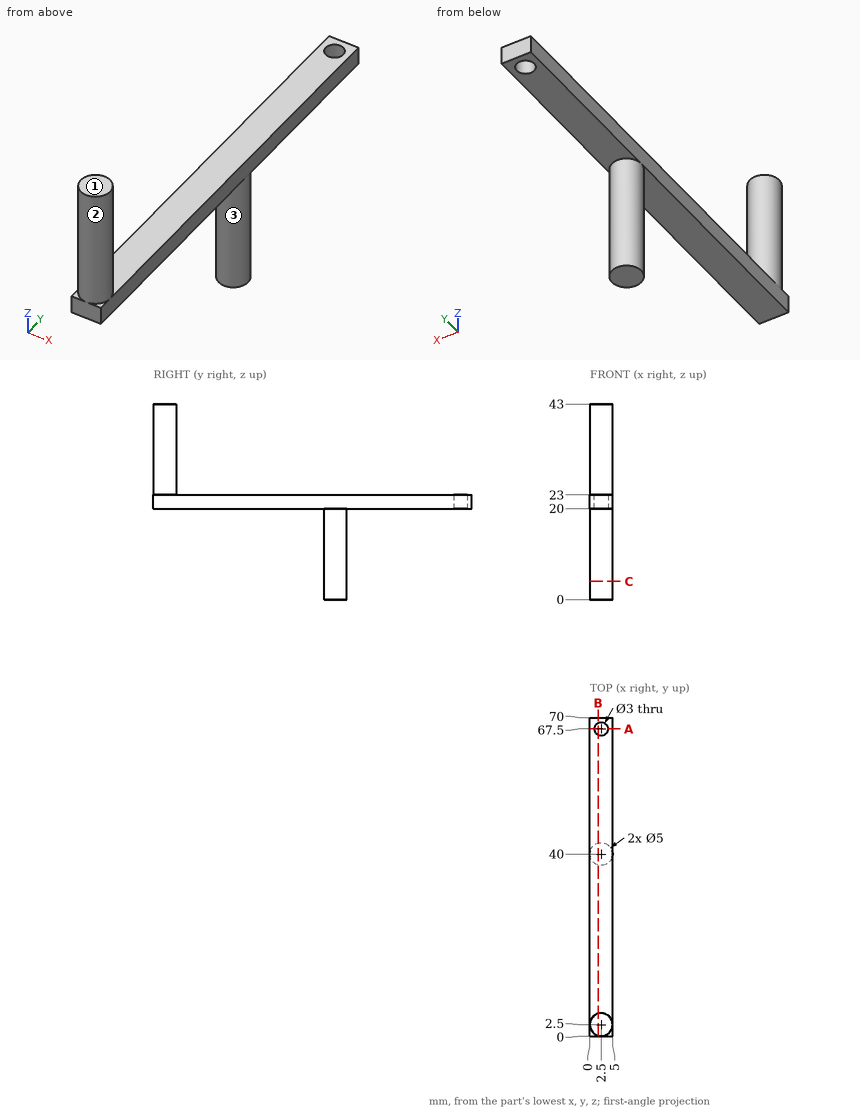
Part print with two shaded views. Sizes in mm from the minimum x, y, z corner. A direction names the side the tool comes from. Coordinates: 2 decimals unless noted, no trailing zeros. Write each loop counter-clockwise with the first axis right and the second up, starting at its lowest first coordinate (ties: lowest second). Pieces come first, ordered by that corner, then holes. Notation, with made-up numbers: (14.25, -37.75) - (69.25, -37.75) arc R24 ccw to (69.25, -27.75) - close; hole circle Ø7 at (89.25, -15.5). An arc over 180 degrees is marked (long way). One line per item, written item: value. Start each with the question number.
1. Slice it at B-B (x = 1.8). Write the cut outline in (y, z).
2. Flat gauge pins, fed straight in: pin 1 (1.5 mm diameter, centred on x = 3.5, y = 26.5, fed in from -Z); pin 2 (1.5 mm diameter, centred on x = 3.5, y = 45, fed in from +Z). Where does each tip first touch, or does it go through?
3. Tool access for the marked faces 1, 2 and 3: list every direction of +Z, -Z, +X, -X, +Y, -Y with a clear straight run to the whole face (end or side of a thin tool).
4. Slice it at A-A (y = 67.5). Write the cut outline in (x, z).
5. Probe line 1 (Y direction, x = 2.5, z = 21.1); line 2 (X direction, y = 67.5, z = 21.25); line 3 (Z direction, x = 2.95, y = 60). List the from-to ranges inside material, lowest first. Write a range as from..to.
6. Slice it at C-C (z = 4). Write the cut outline in (x, y).
Answers below:
1. outline: (0, 20) - (37.6, 20) - (37.6, 0) - (42.4, 0) - (42.4, 20) - (66.17, 20) - (66.17, 23) - (4.9, 23) - (4.9, 43) - (0.1, 43) - (0.1, 23) - (0, 23) - close; (68.83, 20) - (70, 20) - (70, 23) - (68.83, 23) - close
2. pin 1: stops at z = 20
2. pin 2: stops at z = 23
3. face 1: +Z, +X, -X, +Y, -Y
3. face 2: +Z
3. face 3: -Z
4. outline: (0, 20) - (1, 20) - (1, 23) - (0, 23) - close; (4, 20) - (5, 20) - (5, 23) - (4, 23) - close
5. line 1: y = 0..66, 69..70
5. line 2: x = 0..1, 4..5
5. line 3: z = 20..23
6. outline: circle Ø5 at (2.5, 40)
